Verification items for the finished model (mm, model axes). A direction names the side the tool comes from. Coordinates: 2 decimals unless noted, no trailing zeros. Order: outer loops, then holes, each group sorted by start corner. A loop starts at its lowest first (then second) coordinate and runs counter-clockwise, first axis right, second up. Notation, with made-up numbers: M 47,66 L 71,66 A21 cw 71,103 Z; hole C 73,-40 d6. An arc over 180 degrees is marked long. Write item = value, one per line.
```python
from build123d import *

# Parameters (mm, degrees)
F0_R     = 1.6
F1_DEPTH = 2
F3_DEPTH = 2.001
F5_DEPTH = 1
F6_R     = 0.5


with BuildPart() as f1:
    # F0 (on Front) → F1 (new body)
    with BuildSketch(Plane.XZ):
        with BuildLine():
            ThreePointArc((0, 4.5), (1.318019, 1.318019), (4.5, 0))
            Line((4.5, 0), (39.5, 0))
            ThreePointArc((39.5, 0), (42.681981, 1.318019), (44, 4.5))
            Line((44, 4.5), (44, 13.136039))
            ThreePointArc((44, 13.136039), (43.657458, 14.858114), (42.681981, 16.318019))
            Line((42.681981, 16.318019), (29.5, 29.5))
            Line((29.5, 29.5), (16.318019, 42.681981))
            ThreePointArc((16.318019, 42.681981), (14.858114, 43.657458), (13.136039, 44))
            Line((13.136039, 44), (4.5, 44))
            ThreePointArc((4.5, 44), (1.318019, 42.681981), (0, 39.5))
            Line((0, 39.5), (0, 4.5))
        make_face()
        with Locations((7, 7)):
            Circle(F0_R, mode=Mode.SUBTRACT)
        with Locations((22, 7)):
            Circle(F0_R, mode=Mode.SUBTRACT)
        with Locations((37, 7)):
            Circle(F0_R, mode=Mode.SUBTRACT)
        with Locations((7, 22)):
            Circle(F0_R, mode=Mode.SUBTRACT)
        with Locations((7, 37)):
            Circle(F0_R, mode=Mode.SUBTRACT)
        with Locations((22, 22)):
            Circle(F0_R, mode=Mode.SUBTRACT)
    extrude(amount=F1_DEPTH)

    # F2 (on Front) → F3 (cut, through all)
    with BuildSketch(Plane.XZ):
        with BuildLine():
            ThreePointArc((31.20675, 13.772435), (33.054509, 15.007068), (32.620963, 17.186649))
            Line((32.620963, 17.186649), (30.220545, 19.587067))
            ThreePointArc((30.220545, 19.587067), (27.880232, 20.457743), (25.691636, 19.255583))
            ThreePointArc((25.691636, 19.255583), (23.783316, 17.759743), (21.379509, 17.442041))
            ThreePointArc((21.379509, 17.442041), (20.016778, 17.312365), (18.853521, 16.590779))
            Line((18.853521, 16.590779), (17.742284, 15.479542))
            ThreePointArc((17.742284, 15.479542), (17.525511, 14.389752), (18.44939, 13.772435))
            Line((18.44939, 13.772435), (31.20675, 13.772435))
        make_face()
        with BuildLine():
            ThreePointArc((16.590779, 18.853521), (17.312365, 20.016778), (17.442041, 21.379509))
            ThreePointArc((17.442041, 21.379509), (17.759743, 23.783316), (19.255583, 25.691636))
            ThreePointArc((19.255583, 25.691636), (20.457743, 27.880232), (19.587067, 30.220545))
            Line((19.587067, 30.220545), (17.186649, 32.620963))
            ThreePointArc((17.186649, 32.620963), (15.007068, 33.054509), (13.772435, 31.20675))
            Line((13.772435, 31.20675), (13.772435, 18.44939))
            ThreePointArc((13.772435, 18.44939), (14.389752, 17.525511), (15.479542, 17.742284))
            Line((15.479542, 17.742284), (16.590779, 18.853521))
        make_face()
    extrude(amount=F3_DEPTH, mode=Mode.SUBTRACT)

    # F4 (on face) → F5 (join)
    with BuildSketch(Plane.XZ.offset(2)):
        with BuildLine():
            Line((0, 39.5), (0, 4.5))
            ThreePointArc((0, 4.5), (1.318019, 1.318019), (4.5, 0))
            Line((4.5, 0), (39.5, 0))
            ThreePointArc((39.5, 0), (42.681981, 1.318019), (44, 4.5))
            Line((44, 4.5), (44, 13.136039))
            ThreePointArc((44, 13.136039), (43.657458, 14.858114), (42.681981, 16.318019))
            Line((42.681981, 16.318019), (29.5, 29.5))
            Line((29.5, 29.5), (16.318019, 42.681981))
            ThreePointArc((16.318019, 42.681981), (14.858114, 43.657458), (13.136039, 44))
            Line((13.136039, 44), (4.5, 44))
            ThreePointArc((4.5, 44), (1.318019, 42.681981), (0, 39.5))
        make_face()
        with BuildLine():
            ThreePointArc((41.62132, 15.257359), (42.271639, 14.284089), (42.5, 13.136039))
            Line((42.5, 13.136039), (42.5, 4.5))
            ThreePointArc((42.5, 4.5), (41.62132, 2.37868), (39.5, 1.5))
            Line((39.5, 1.5), (4.5, 1.5))
            ThreePointArc((4.5, 1.5), (2.37868, 2.37868), (1.5, 4.5))
            Line((1.5, 4.5), (1.5, 39.5))
            ThreePointArc((1.5, 39.5), (2.37868, 41.62132), (4.5, 42.5))
            Line((4.5, 42.5), (13.136039, 42.5))
            ThreePointArc((13.136039, 42.5), (14.284089, 42.271639), (15.257359, 41.62132))
            Line((15.257359, 41.62132), (28.43934, 28.43934))
            Line((28.43934, 28.43934), (41.62132, 15.257359))
        make_face(mode=Mode.SUBTRACT)
    extrude(amount=F5_DEPTH)

    # F6
    f6_edges = [f1.edges().sort_by_distance(p)[0] for p in [
        (1.5, -3, 22),
        (0, -3, 22),
        (20.016778, -2, 17.312365),
        (17.312365, -2, 20.016778),
    ]]
    fillet(f6_edges, radius=F6_R)


solid = f1.part
```
Item 1: Sectioned sample at A-A, the plane z = 7. Enter the section's corners in (x, y).
Report:
outline = M 0,-2.5 A0.5 ccw 0.5,-3 L 1,-3 A0.5 ccw 1.5,-2.5 L 1.5,-2 L 5.4,-2 L 5.4,0 L 0,0 Z; M 8.6,-2 L 20.4,-2 L 20.4,0 L 8.6,0 Z; M 23.6,-2 L 35.4,-2 L 35.4,0 L 23.6,0 Z; M 38.6,-2 L 42.5,-2 L 42.5,-2.5 A0.5 ccw 43,-3 L 43.5,-3 A0.5 ccw 44,-2.5 L 44,0 L 38.6,0 Z
Item 2: Tool access check on faces 4 (the cylindrical face through (1.353, -1.232, 42.717)), 5 (the cylindrical face through (27.92, -0.74, 20.46)), 6 (the cylindrical face through (41.64, -2.25, 2.4)). Record the directions out of +Z, -Z, +X, -X, +Y, -Y that give a thin tool (end or side, any length) a straight path to the whole face; none if there is none.
Report:
face_4 = +Z, -X, +Y, -Y
face_5 = +Y, -Y
face_6 = -Y
Item 3: Gauge pin test, flat ends, axial feed: pin 1 (3.5 mm diameter, centred on x = 22, z = 7, fed in from -Y); pin 2 (2.5 mm diameter, centred on x = 22, z = 22, fed in from +Y); pin 3 (1 mm diameter, centred on y = -2, z = 20.5, fed in from +X); pin 4 (1.2 mm diameter, centred on y = -1, z = 24.5, fed in from +X). Record the tip position at first contact, or that the pin passes through.
Report:
pin_1 = -2
pin_2 = through
pin_3 = 39
pin_4 = 35.1
Item 4: Scan lines: L1, parallel to Z at x = 7, y = -0.95; L2, parallel to Z at x = 19, y = -0.2; L3, parallel to Y at x = 34.5, z = 9. Record each from-to range of solid material in increasing order. Write a range as from..to.
Report:
L1 = 0..5.4, 8.6..20.4, 23.6..35.4, 38.6..44
L2 = 0..13.77, 16.73..25.49, 30.81..40
L3 = -2..0
Item 5: Release check for a two-part mould opening along X. For faces 1 (the cylindrical face through (2.36, -2.25, 41.6)), 2 (the flat face through (30, -1, 29)), 3 (the flat face through (9, -1, 44)) record: pulls with the +X half, pulls with the -X half, needs draft (parallel to the pull), parting line crosses it, or undercut.
Report:
face_1 = undercut
face_2 = pulls with the +X half
face_3 = needs draft
Item 6: Sectioned sample at D-D, the plane y = -0.5. Give the number of separate pieces and of enclosed holes in the cut face, then the cut area to 3 significant figures.
Report:
separate_pieces = 1
enclosed_holes = 8
area = 1,310 mm^2
Item 7: Sectioned sample at B-B, the plane x = 7. Enter the section's corners in (y, z).
Report:
outline = M -3,0.5 A0.5 ccw -2.5,0 L 0,0 L 0,5.4 L -2,5.4 L -2,1.5 L -2.5,1.5 A0.5 ccw -3,1 Z; M -3,43 A0.5 ccw -2.5,42.5 L -2,42.5 L -2,38.6 L 0,38.6 L 0,44 L -2.5,44 A0.5 ccw -3,43.5 Z; M -2,8.6 L 0,8.6 L 0,20.4 L -2,20.4 Z; M -2,23.6 L 0,23.6 L 0,35.4 L -2,35.4 Z
Item 8: Sectioned sample at C-C, the plane z = 12. Enter the section's corners in (x, y), then the cut area to 3 significant figures.
Report:
outline = M 0,-2.5 A0.5 ccw 0.5,-3 L 1,-3 A0.5 ccw 1.5,-2.5 L 1.5,-2 L 42.5,-2 L 42.5,-2.5 A0.5 ccw 43,-3 L 43.5,-3 A0.5 ccw 44,-2.5 L 44,0 L 0,0 Z
area = 90.8 mm^2
